Build history of the part. All positions in model axes, mm. Round coordinates to 2 decimals unless told otherwise and drop trailing zeros. Write each loop counter-clockwise with the first axis right and the second up, starting at its lowest first coordinate (ties: lowest second). Pieces come first, ordered by that corner, then holes.
1) Wall check: probe 1 along X at (y, z) = (36, 0.6); probe 2 along X at (y, z) = (5, 1.65) (3 decimals); probe 3 along Y at (x, z) = (50, 0.9). Give the ranges that are in metal, low to high.
2) Saw through at C-C (y = 31). Write the cut outline in (x, z), plus the area to 3 significant figures.
3) Flat gauge pins, fed straight in: pin 1 (1.6 mm diameter, centred on x = 62, z = 2, fed in from -Y); pin 2 (0.9 mm diameter, centred on x = 53, z = 1.5, fed in from +Y); pin 3 (1.6 mm diameter, centred on y = 37, z = 1.5, fed in from -X). Where does each tip first touch, or does it go through?
4) Saw through at A-A (z = 0.8). Write the cut outline in (x, y) (3 decimals).
5) Saw through at B-B (x = 48). Write the cut outline in (y, z).
Autodesk Inventor part; units mm, degrees
ref_plane "YZ Plane" through (0, 0, 0) normal (1, 0, 0) x (0, 1, 0)
ref_plane "XZ Plane" through (0, 0, 0) normal (0, 1, 0) x (-1, 0, 0)
ref_plane "XY Plane" through (0, 0, 0) normal (0, 0, 1) x (1, 0, 0)
sketch "Sketch1" plane through (0, 0, 0) normal (0, 0, 1) x (1, 0, 0)
  line L0 (0, 0) -> (127, 0)
  line L1 (127, 0) -> (127, 76.2)
  line L2 (127, 76.2) -> (0, 76.2)
  line L3 (0, 76.2) -> (0, 0)
  dimension "d0" = 127
  dimension "d1" = 76.2
extrude "Extrusion1" add sketch "Sketch1" along normal blind 3.1496
sketch "Sketch4" plane through (0, 0, 3.1496) normal (0, 0, 1) x (1, 0, 0)
  line L0 (0, 0) -> (127, 0)
  line L1 (127, 0) -> (127, 76.2)
  line L2 (127, 76.2) -> (0, 76.2)
  line L3 (0, 76.2) -> (0, 0)
  line L4 (0, 50.8) -> (3.1496, 50.8)
  line L5 (3.1496, 50.8) -> (3.1496, 25.4)
  line L6 (3.1496, 25.4) -> (0, 25.4)
  line L7 (0, 25.4) -> (0, 50.8)
  line L8 (127, 50.8) -> (123.8504, 50.8)
  line L9 (123.8504, 50.8) -> (123.8504, 25.4)
  line L10 (123.8504, 25.4) -> (127, 25.4)
  line L11 (127, 25.4) -> (127, 50.8)
  line L12 (42.3333, 76.2) -> (84.6667, 76.2)
  line L13 (84.6667, 76.2) -> (84.6667, 73.0504)
  line L14 (84.6667, 73.0504) -> (42.3333, 73.0504)
  line L15 (42.3333, 73.0504) -> (42.3333, 76.2)
  dimension "d7" = 3.1496
  dimension "d8" = 25.4
  dimension "d9" = 25.4
  dimension "d10" = 3.1496
  dimension "d11" = 25.4
  dimension "d12" = 25.4
  dimension "d13" = 42.3333
  dimension "d14" = 3.1496
  dimension "d15" = 42.3333
extrude "Extrusion2" cut sketch "Sketch4" against normal blind 3.1496 contours L3 L4 L5 L6 | L10 L9 L8 L1 | L2 L13 L14 L15
sketch "Sketch5" plane through (0, 0, 3.1496) normal (0, 0, 1) x (1, 0, 0)
  line L0 (0, 25.4) -> (0, 0)
  line L1 (0, 0) -> (127, 0)
  line L2 (60.325, 0) -> (66.675, 0)
  line L3 (66.675, 0) -> (66.675, 6.35)
  line L4 (66.675, 6.35) -> (60.325, 6.35)
  line L5 (60.325, 6.35) -> (60.325, 0)
  dimension "d18" = 6.35
  dimension "d19" = 6.35
  dimension "d20" = 60.325
extrude "Extrusion3" cut sketch "Sketch5" against normal blind 3.1496
equation "\"d0\" = width"
equation "\"d1\" = height"
equation "\"d2\" = thick"
equation "\"d7\" = thick"
equation "\"d8\" = 0.333333 * height"
equation "\"d9\" = 0.333333 * height"
equation "\"d10\" = thick"
equation "\"d11\" = 0.333333 * height"
equation "\"d12\" = 0.333333 * height"
equation "\"d13\" = 0.333333 * width"
equation "\"d14\" = thick"
equation "\"d15\" = 0.333333 * width"
equation "\"d16\" = thick"
equation "\"d21\" = thick"
equation "\"height\" = 76.2"
equation "\"width\" = 127"
equation "\"thick\" = 3.1496"
properties part number "Front"
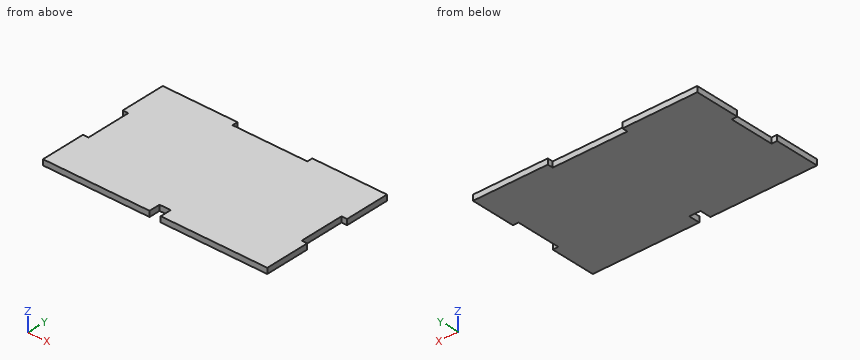
Evaluation:
1. probe 1: x = 3.15 to 123.85
1. probe 2: x = 0 to 60.325, 66.675 to 127
1. probe 3: y = 0 to 73.05
2. outline: (3.15, 0) - (123.85, 0) - (123.85, 3.15) - (3.15, 3.15) - close
2. area: 380 mm2
3. pin 1: stops at y = 6.35
3. pin 2: stops at y = 73.05
3. pin 3: stops at x = 3.15
4. outline: (0, 0) - (60.325, 0) - (60.325, 6.35) - (66.675, 6.35) - (66.675, 0) - (127, 0) - (127, 25.4) - (123.85, 25.4) - (123.85, 50.8) - (127, 50.8) - (127, 76.2) - (84.667, 76.2) - (84.667, 73.05) - (42.333, 73.05) - (42.333, 76.2) - (0, 76.2) - (0, 50.8) - (3.15, 50.8) - (3.15, 25.4) - (0, 25.4) - close
5. outline: (0, 0) - (73.05, 0) - (73.05, 3.15) - (0, 3.15) - close
